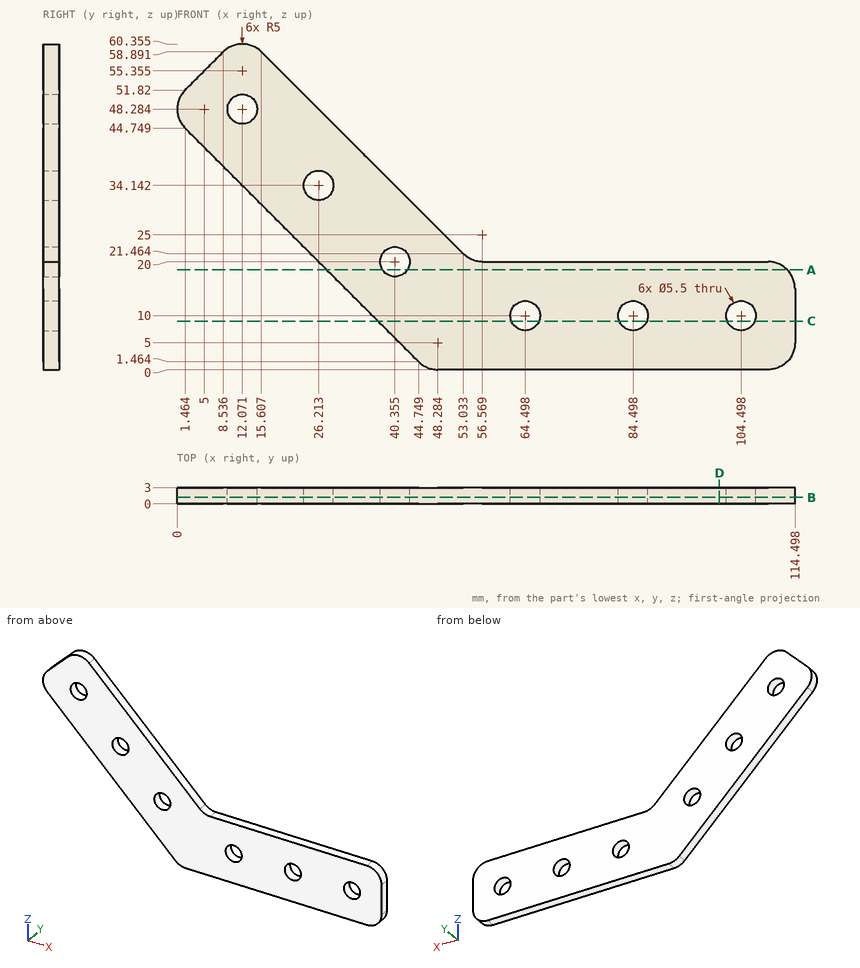
The figure shows three views and two pictorial views of one solid part (mm, origin at its lowest corner). Answer the questions. Coordinates: 2 decimals unless noted, no trailing zeros. Loops run counter-clockwise (first coordinate to the right, second up) from the corner with the lowest first, then second, coordinate; pieces in that order, holes last.
1) Find section B-B on y = 1.2. Give the number of separate pieces and of enclosed holes in the cut face, then the cut area to 3 significant figures.
2) Find section C-C on z = 9. Write down the section's boundary in (x, y) (1 decimal), then the cut area to 3 significant figures.
3) Find the intervals of material crossed by L1, parallel to Z at x = 109, y = 0.9; L2, parallel to Z at x = 105, y = 0.85 (1 decimal); L3, parallel to Z at x = 40.5, y = 0.75 (1 decimal), in increasing order.
4) Find section D-D on x = 100.5. Write down the section's boundary in (y, z), then the cut area to 3 significant figures.
5) Find section A-A on z = 18.5. Write down the section's boundary in (x, y).
6) A flat-ended cylindrical pin translates along its axis: pin 1 Ø3.5 at (x, z) = (104.5, 10) entering from -Y. Find the tip coordinate at first contact, or state that the pin passes through.
Values:
1. separate pieces: 1
1. enclosed holes: 6
1. area: 2,400 mm2
2. outline: (37.2, 0) - (61.9, 0) - (61.9, 3) - (37.2, 3) - close; (67.1, 0) - (81.9, 0) - (81.9, 3) - (67.1, 3) - close; (87.1, 0) - (101.9, 0) - (101.9, 3) - (87.1, 3) - close; (107.1, 0) - (114.5, 0) - (114.5, 3) - (107.1, 3) - close
2. area: 186 mm2
3. L1: z = 0 to 20
3. L2: z = 0 to 7.3, 12.7 to 20
3. L3: z = 5.7 to 17.3, 22.7 to 34
4. outline: (0, 0) - (3, 0) - (3, 20) - (0, 20) - close
4. area: 60.0 mm2
5. outline: (27.71, 0) - (38.05, 0) - (38.05, 3) - (27.71, 3) - close; (42.66, 0) - (113.07, 0) - (113.07, 3) - (42.66, 3) - close
6. pin 1: passes through
